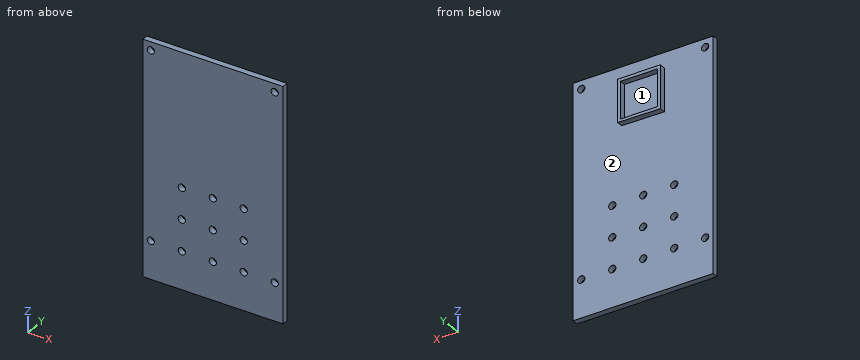
Autodesk Inventor part; units mm, degrees
ref_plane "YZ Plane" through (0, 0, 0) normal (1, 0, 0) x (0, 1, 0)
ref_plane "XZ Plane" through (0, 0, 0) normal (0, 1, 0) x (-1, 0, 0)
ref_plane "XY Plane" through (0, 0, 0) normal (0, 0, 1) x (1, 0, 0)
sketch "스케치1" plane through (0, 0, 0) normal (0, 1, 0) x (-1, 0, 0)
  line L0 (0, 0) -> (-115, 0)
  line L1 (-115, 0) -> (-115, -190)
  line L2 (-115, -190) -> (0, -190)
  line L3 (0, -190) -> (0, 0)
  circle A0 centre (-6.5, -6.8) radius 2.95
  line L4 (0, -95) -> (-115, -95) construction
  line L5 (-57.5, 0) -> (-57.5, -190) construction
  circle A1 centre (-6.5, -183.2) radius 2.95
  circle A2 centre (-6.5, -32.2) radius 2.95
  circle A3 centre (-6.5, -57.6) radius 2.95
  circle A4 centre (-6.5, -83) radius 2.95
  circle A5 centre (-6.5, -108.4) radius 2.95
  circle A6 centre (-6.5, -133.8) radius 2.95
  circle A7 centre (-6.5, -159.2) radius 2.95
  circle A8 centre (-31.9, -6.8) radius 2.95
  circle A9 centre (-31.9, -32.2) radius 2.95
  circle A10 centre (-31.9, -57.6) radius 2.95
  circle A11 centre (-31.9, -83) radius 2.95
  circle A12 centre (-31.9, -108.4) radius 2.95
  circle A13 centre (-31.9, -133.8) radius 2.95
  circle A14 centre (-31.9, -159.2) radius 2.95
  circle A15 centre (-57.3, -6.8) radius 2.95
  circle A16 centre (-57.3, -32.2) radius 2.95
  circle A17 centre (-57.3, -57.6) radius 2.95
  circle A18 centre (-57.3, -83) radius 2.95
  circle A19 centre (-57.3, -108.4) radius 2.95
  circle A20 centre (-57.3, -133.8) radius 2.95
  circle A21 centre (-57.3, -159.2) radius 2.95
  circle A22 centre (-82.7, -6.8) radius 2.95
  circle A23 centre (-82.7, -32.2) radius 2.95
  circle A24 centre (-82.7, -57.6) radius 2.95
  circle A25 centre (-82.7, -83) radius 2.95
  circle A26 centre (-82.7, -108.4) radius 2.95
  circle A27 centre (-82.7, -133.8) radius 2.95
  circle A28 centre (-82.7, -159.2) radius 2.95
  circle A29 centre (-108.1, -6.8) radius 2.95
  circle A30 centre (-108.1, -32.2) radius 2.95
  circle A31 centre (-108.1, -57.6) radius 2.95
  circle A32 centre (-108.1, -83) radius 2.95
  circle A33 centre (-108.1, -108.4) radius 2.95
  circle A34 centre (-108.1, -133.8) radius 2.95
  circle A35 centre (-108.1, -159.2) radius 2.95
  circle A36 centre (-133.5, -6.8) radius 2.95
  circle A37 centre (-133.5, -32.2) radius 2.95
  circle A38 centre (-133.5, -57.6) radius 2.95
  circle A39 centre (-133.5, -83) radius 2.95
  circle A40 centre (-133.5, -108.4) radius 2.95
  circle A41 centre (-133.5, -133.8) radius 2.95
  circle A42 centre (-133.5, -159.2) radius 2.95
  dimension "d0" = 190
  dimension "d1" = 115
  dimension "d2" = 6.5
  dimension "d3" = 6.8
  dimension "d4" = 5.9
  dimension "d9" = 25.4
  dimension "d12" = 25.4
extrude "돌출1" add sketch "스케치1" along normal blind 5 contours L3 L2 L1 L0 | A1 | A2 | A3 | A4 | A5 | A6 | A7 | A8 | A9 | A10 | A11 | A12 | A13 | A14 | A15 | A16 | A17 | A18 | A19 | A20 | A21 | A22 | A23 | A24 | A25 | A26 | A27 | A28 | A29 | A30 | A31 | A32 | A33 | A34 | A35
extrude "돌출2" cut sketch "스케치1" along normal blind 5 contours A12 | A13 | A14 | A19 | A20 | A21 | A26 | A27 | A28
extrude "돌출4" cut sketch "스케치1" along normal blind 5 contours A35
extrude "돌출5" cut sketch "스케치1" along normal blind 5 contours A7
sketch "스케치2" plane through (0, 5, 0) normal (0, 1, 0) x (1, 0, 0)
  circle A0 centre (57.5, 63.8) radius 2.5
  line L0 (0, 0) -> (115, 0)
  circle A1 centre (57.3, 133.8) radius 2.95
  point P0 (57.5, 0)
  dimension "d23" = 70
  dimension "d24" = 5
extrude "돌출6" cut sketch "스케치1" along normal blind 5 contours A29
sketch "스케치3" plane through (0, 5, 0) normal (0, 1, 0) x (1, 0, 0)
  line L0 (42.4, 14.8) -> (72.6, 14.8)
  line L1 (72.6, 14.8) -> (72.6, 45)
  line L2 (72.6, 45) -> (42.4, 45)
  line L3 (42.4, 45) -> (42.4, 14.8)
  line L4 (115, 190) -> (0, 190)
  line L5 (40.0511, 12.35) -> (74.9489, 12.35)
  line L6 (74.9489, 12.35) -> (74.9489, 47.05)
  line L7 (74.9489, 47.05) -> (40.0511, 47.45)
  line L8 (40.0511, 47.45) -> (40.0511, 12.35)
  line L9 (0, 0) -> (115, 0)
  point P0 (57.5, 45)
  point P1 (57.5, 190)
  point P2 (57.5, 190)
  point P3 (57.5, 47.25)
  point P4 (57.5, 12.35)
  point P5 (40.0511, 29.9)
  point P6 (42.4, 29.9)
  dimension "d27" = 30.2
  dimension "d28" = 30.2
  dimension "d29" = 145
  dimension "d31" = 34.9
  dimension "d34" = 2.45
  dimension "d35" = 34.9
extrude "돌출7" add sketch "스케치3" along normal blind 5
properties part number "mounting_board_printed"
Check sheet for the modelled part. Datum: model origin and axes. Units: mm. Face numbers are marked on the shaded views. Round coordinates to 2 decimals unless told otherwise and drop trailing zeros. Order: outer loops, then holes, each group sorted by start corner. A loop starts at its lowest first (then second) coordinate and runs counter-clockwise, first axis right, second up. Notation, with made-up numbers: (3, 75) -> (55, 75) arc R18 ccw to (55, 106) -> close; hole circle Ø3 at (55.5, 51.5). An arc over 180 degrees is marked (long way). Use CSV: the item, a comma, the result in double quotes.
(1) Cross-section at A-A (z = -6.8). Record the boundary of the cut face in (x, y), and give its area (3 significant figures).
Worked out:
outline,"(0, 0) -> (3.55, 0) -> (3.55, 5) -> (0, 5) -> close; (9.45, 0) -> (105.15, 0) -> (105.15, 5) -> (9.45, 5) -> close; (111.05, 0) -> (115, 0) -> (115, 5) -> (111.05, 5) -> close"
area,"516 mm²"
(2) Material ranges on line 1 along Z through (x, y) = (6.5, 3.2); line 2 along Z through (x, y) = (31.9, 2.7); line 3 along X through (y, z) = (3.25, -133.8), recorded low to high. Write a range as from..to.
Worked out:
line 1,"-190..-162.15, -156.25..-9.75, -3.85..0"
line 2,"-190..-162.15, -156.25..-136.75, -130.85..-111.35, -105.45..0"
line 3,"0..28.95, 34.85..54.35, 60.25..79.75, 85.65..115"
(3) Cross-section at D-D (x = 6.5). Record the boundary of the cut face in (y, z).
Worked out:
outline,"(0, -190) -> (5, -190) -> (5, -162.15) -> (0, -162.15) -> close; (0, -156.25) -> (5, -156.25) -> (5, -9.75) -> (0, -9.75) -> close; (0, -3.85) -> (5, -3.85) -> (5, 0) -> (0, 0) -> close"
(4) Cross-section at B-B (y = 6.5). Record the boundary of the cut face in (x, z), and give its area (3 significant figures).
Worked out:
outline,"(40.05, -47.45) -> (74.95, -47.05) -> (74.95, -12.35) -> (40.05, -12.35) -> close; hole (42.4, -45) -> (72.6, -45) -> (72.6, -14.8) -> (42.4, -14.8) -> close"
area,"306 mm²"
(5) Cross-section at C-C (x = 31.9). Record the boundary of the cut face in (y, z).
Worked out:
outline,"(0, -190) -> (5, -190) -> (5, -162.15) -> (0, -162.15) -> close; (0, -156.25) -> (5, -156.25) -> (5, -136.75) -> (0, -136.75) -> close; (0, -130.85) -> (5, -130.85) -> (5, -111.35) -> (0, -111.35) -> close; (0, -105.45) -> (5, -105.45) -> (5, 0) -> (0, 0) -> close"
(6) Draft check along Z on the marked faces 1 and 2. Enter one of: pulls with the +Z half, pulls with the -Z half, needs draft (parallel to the pull), parting line crosses it, or undercut.
Worked out:
face 1,"undercut"
face 2,"needs draft"
(7) Depth check by flat-ended pin: pin 1 (1.5 mm diameter, centred on y = 7.5, z = -164.5, fed in from +X); pin 2 (1.5 mm diameter, centred on y = 6.5, z = -34, fed in from -X); pin 3 (9.5 mm diameter, centred on x = 6.5, z = -6.8, fed in from +Y); pin 4 (5.5 mm diameter, centred on x = 56, y = 8.5, fed in from +Z). Enter the tip coordinate at first touch or a pass-through.
Worked out:
pin 1,"through"
pin 2,"x = 40.05"
pin 3,"y = 5"
pin 4,"z = -12.35"
